The model under review builds one solid part; all positions refer to its coordinate system, in mm. A direction names the side the tool comes from. Coordinates: 2 decimals unless noted, no trailing zeros. Order: outer loops, then holes, each group sorted by start corner. A loop starts at its lowest first (then second) coordinate and runs counter-clockwise, first axis right, second up. Notation, with made-up numbers: (25.5, -14) -> (50.5, -14) arc R9 cw to (50.5, -3) -> close; hole circle Ø11 at (44, 60.5). An arc over 180 degrees is marked (long way). Put each result on its own line as item: value.
from build123d import *

# Parameters (mm, degrees)
SKETCH_1_W                       = 35
SKETCH_1_H                       = 44
EXTRUDE_1_DEPTH                  = 30.5
SKETCH_3_W                       = 41
SKETCH_3_H                       = 40
CUT_EXTRUDE_1_DEPTH              = 33
SKETCH_4_W                       = 41
SKETCH_4_H                       = 12
CUT_EXTRUDE_2_DEPTH              = 33
SKETCH_5_R                       = 8
CUT_EXTRUDE_3_DEPTH              = 83.957820608
HOLE_WIZARD_6_5_6_5_1_AT_2_COUNT = 2
HOLE_WIZARD_6_5_6_5_1_AT_2_PITCH = 18


# Read off the part's stored shape, not the designer's step: M1.6 螺纹孔1, M6 螺纹孔1
with BuildPart() as part:
    # 草图1 → 凸台-拉伸1 (new, symmetric)
    with BuildSketch(Plane.XY):
        with Locations((17.5, 22)):
            Rectangle(SKETCH_1_W, SKETCH_1_H)
    extrude(amount=EXTRUDE_1_DEPTH, both=True)

    # 草图3 → 切除-拉伸1 (cut)
    with BuildSketch(Plane(origin=(35, 0, 0), x_dir=(0, 0, -1), z_dir=(1, 0, 0))):
        with Locations((0, 24)):
            Rectangle(SKETCH_3_W, SKETCH_3_H)
    extrude(amount=-CUT_EXTRUDE_1_DEPTH, mode=Mode.SUBTRACT)

    # 草图4 → 切除-拉伸2 (cut)
    with BuildSketch(Plane(origin=(2, 0, 0), x_dir=(0, 0, -1), z_dir=(1, 0, 0))):
        with Locations((0, 38)):
            Rectangle(SKETCH_4_W, SKETCH_4_H)
    extrude(amount=-CUT_EXTRUDE_2_DEPTH, mode=Mode.SUBTRACT)

    # 草图5 → 切除-拉伸3 (cut, through all)
    with BuildSketch(Plane.XY.offset(30.5)):
        with Locations((10.5, 14)):
            Circle(SKETCH_5_R)
    extrude(amount=-CUT_EXTRUDE_3_DEPTH, mode=Mode.SUBTRACT)

    # 草图7 → Ø6.5 (6.5) 直径孔1 (revolve, cut)
    with BuildSketch(Plane(origin=(9, 38, -20.5), x_dir=(0, -1, 0), z_dir=(1, 0, 0))):
        Polygon((0, 0), (0, 10), (5.25, 10), (3.25, 8), (3.25, 0), align=None)
    hole_wizard_6_5_6_5_1 = revolve(axis=Axis((9, 38, -14.15), (0, 0, -1)), mode=Mode.SUBTRACT)

    # Ø6.5 (6.5) 直径孔1 at 2: Ø6.5 (6.5) 直径孔1 ×2
    with Locations(*[(i * HOLE_WIZARD_6_5_6_5_1_AT_2_PITCH, 0, 0) for i in range(1, HOLE_WIZARD_6_5_6_5_1_AT_2_COUNT)]):
        add(hole_wizard_6_5_6_5_1, mode=Mode.SUBTRACT)

    # 镜向1: Ø6.5 (6.5) 直径孔1 across plane
    add(hole_wizard_6_5_6_5_1.mirror(Plane.XY), mode=Mode.SUBTRACT)

    # 镜向1 copy 1 sketch → 镜向1 copy 1 (revolve, cut)
    with BuildSketch(Plane(origin=(27, 38, 20.5), x_dir=(0, -1, 0), z_dir=(1, 0, 0))):
        Polygon((0, 0), (0, -10), (5.25, -10), (3.25, -8), (3.25, 0), align=None)
    revolve(axis=Axis((27, 38, 14.15), (0, 0, -1)), mode=Mode.SUBTRACT)

    # M1.6 螺纹孔1 outline → M1.6 螺纹孔1 (revolve, cut)
    with BuildSketch(Plane(origin=(0, 27.5, 25.5), x_dir=(0, 1, 0), z_dir=(0, 0, -1))):
        Polygon((0, 35), (0, 26.624462113), (0.625, 27), (0.625, 35), align=None)
    revolve(axis=Axis((0, 27.5, 25.5), (1, 0, 0)), mode=Mode.SUBTRACT)

    # Hole Wizard M1.6 _1 2 outline → Hole Wizard M1.6 _1 2 (revolve, cut)
    with BuildSketch(Plane(origin=(0, 4.5, -24.5), x_dir=(0, 1, 0), z_dir=(0, 0, -1))):
        Polygon((0, 35), (0, 26.624462113), (0.625, 27), (0.625, 35), align=None)
    revolve(axis=Axis((0, 4.5, -24.5), (1, 0, 0)), mode=Mode.SUBTRACT)

    # Hole Wizard M1.6 _1 3 outline → Hole Wizard M1.6 _1 3 (revolve, cut)
    with BuildSketch(Plane(origin=(0, 27.5, -24.5), x_dir=(0, 1, 0), z_dir=(0, 0, -1))):
        Polygon((0, 35), (0, 26.624462113), (0.625, 27), (0.625, 35), align=None)
    revolve(axis=Axis((0, 27.5, -24.5), (1, 0, 0)), mode=Mode.SUBTRACT)

    # Hole Wizard M1.6 _1 4 outline → Hole Wizard M1.6 _1 4 (revolve, cut)
    with BuildSketch(Plane(origin=(0, 4.5, 25.5), x_dir=(0, 1, 0), z_dir=(0, 0, -1))):
        Polygon((0, 35), (0, 26.624462113), (0.625, 27), (0.625, 35), align=None)
    revolve(axis=Axis((0, 4.5, 25.5), (1, 0, 0)), mode=Mode.SUBTRACT)

    # M6 螺纹孔1 outline → M6 螺纹孔1 (revolve, cut)
    with BuildSketch(Plane(origin=(0, 14, -25.5), x_dir=(0, 1, 0), z_dir=(0, 0, -1))):
        Polygon((3.025, 2.499998942), (3.025, 3.094213479), (2.5, 3.094219892), (2.5, 1.975), align=None)
        Polygon((2.5, 1.975), (2.5, 3.094219892), (0, 3.094219892), (0, 0), (2.5, 0), align=None)
    revolve(axis=Axis((0, 14, -25.5), (1, 0, 0)), mode=Mode.SUBTRACT)


solid = part.part
Item 1: Consider section B-B on y = 7. Write out the cut boundary in (x, z).
Answers below:
outline: (0, -30.5) -> (6.63, -30.5) -> (6.63, -20.5) -> (2, -20.5) -> (2, 20.5) -> (6.63, 20.5) -> (6.63, 30.5) -> (0, 30.5) -> close; (14.37, -30.5) -> (35, -30.5) -> (35, -20.5) -> (14.37, -20.5) -> close; (14.37, 20.5) -> (35, 20.5) -> (35, 30.5) -> (14.37, 30.5) -> close
Item 2: Consider section C-C on x = 9. Write out the cut boundary in (y, z), and give its area (3 significant figures).
Answers below:
outline: (0, -30.5) -> (6.14, -30.5) -> (6.14, -20.5) -> (4, -20.5) -> (4, 20.5) -> (6.14, 20.5) -> (6.14, 30.5) -> (0, 30.5) -> close; (21.86, -30.5) -> (32.75, -30.5) -> (34.75, -28.5) -> (34.75, -20.5) -> (21.86, -20.5) -> close; (21.86, 20.5) -> (34.75, 20.5) -> (34.75, 28.5) -> (32.75, 30.5) -> (21.86, 30.5) -> close; (41.25, -28.5) -> (43.25, -30.5) -> (44, -30.5) -> (44, -20.5) -> (41.25, -20.5) -> close; (41.25, 20.5) -> (44, 20.5) -> (44, 30.5) -> (43.25, 30.5) -> (41.25, 28.5) -> close
area: 592 mm^2
Item 3: Consider section D-D on z = -1. Write out the cut boundary in (x, y).
Answers below:
outline: (0, 0) -> (35, 0) -> (35, 4) -> (2, 4) -> (2, 32) -> (0, 32) -> close
Item 4: For faces 5 (the flat face through (1, 32, 0)), 6 (the cylindrical face through (2.67, 11.6, -27.34)), 7 (the cylindrical face through (31.06, 4.42, 26.12)), list the 3-axis set-ups (+Z, -Z, +X, -X, +Y, -Y) from which the entire face can be reached by the end or side of a thin tool; tool diameter is ignored.
Answers below:
face 5: +X, -X, +Y
face 6: none
face 7: +X
Item 5: Mouldability with a two-part tool opening along Z and no side actions: class faces 1 (the flat face through (2, 18, 0)), 2 (the cylindrical face through (28.245, 34.998, -24.444)), 3 (the flat face through (17, 22, 30.5)), 4 (the conical face through (26.69, 4.56, -24.41)) as +Z half, -Z half, draft (parallel to the pull), parting line (faces both ways), or undercut.
Answers below:
face 1: undercut
face 2: draft
face 3: +Z half
face 4: undercut
Item 6: Consider section A-A on y = 38. Count the separate pieces of the cut face and the enclosed holes in it, and give its area (3 significant figures).
Answers below:
separate pieces: 6
enclosed holes: 0
area: 424 mm^2
Item 7: For line 1 (Z direction, x = 13, y = 26); line 2 (X direction, y = 38, z = 26.25); line 3 (Y direction, x = 9, z = -24), list the stretches that pass through material, from the lowest coordinate up. Write a range as from..to.
Answers below:
line 1: -30.5..-20.5, 20.5..30.5
line 2: 0..5.75, 12.25..23.75, 30.25..35
line 3: 0..6.14, 21.86..34.75, 41.25..44
Item 8: For pin 1 Ø2 at (x, z) = (0.5, 3.5) entering from +Y; pin 2 Ø14 at (y, z) = (16, -5.5) entering from +X; pin 3 Ø8.5 at (x, y) = (27, 38) entering from -Z; pin 4 Ø9.5 at (x, y) = (10.5, 14) entering from -Z, all flat-tipped, find the tip position at first contact; note any pin that passes through.
Answers below:
pin 1: y = 32
pin 2: x = 2
pin 3: z = -29.5
pin 4: through
